Input: part model. Units: mm. Frame: model coordinates. A direction names the side the tool comes from. Round coordinates to 2 decimals unless told otherwise and drop trailing zeros. Loops run counter-clockwise (first coordinate to the right, second up) from the corner with the lowest first, then second, coordinate; pieces in that order, holes last. Notation, with made-up numbers: M 25.25,78 L 74.25,78 A15 cw 74.25,105 Z; hole C -22.75,17 d10. An arc over 180 degrees is marked long. Return JSON: item names as keys, results as strings. Group by question number.
1) Section C-C (x = 0). Output: boundary loops of the cut face in (y, z).
2) Mould query, pull axis Y, two halves, no side actions, for faces 1 (the face through (-13.851, 17.146, 8.479)), 2 (the face through (-24, 18, 9)), 3 (the face through (19.49, -11.72, 4.93)). Classes: +Y half, -Y half, draft (parallel to the pull), parting line (faces both ways), or undercut.
3) Material intervals for line 1 (Y direction, x = -7, z = 4.5); line 2 (X direction, y = 9, z = 9); line 3 (Y direction, x = -12, z = 3), sorted ascending. Write a range as from..to.
4) Contact query for flat-ended pins moving along their axis: P1, Ø3.5, axis at x = -12, y = 16, coming from the +Z side; P2, Ø1.5, axis at x = -1.5, z = 16.5, coming from the -Y side; P3, Ø12, axis at x = -12.5, z = 11.5, coming from the -Y side; P4, Ø1.5, axis at y = -10.5, z = 6, coming from the -X side. Output: stop coordinate, or through.
5) Section D-D (x = 7.5). Output: boundary loops of the cut face in (y, z).
6) Section A-A (y = 0). Output: boundary loops of the cut face in (x, z).
7) Access query for faces 4 (the face through (13.799, 10.824, 8.479)), 5 (the face through (-0.1, -7.8, 4.9)), 6 (the face through (0, -5, 4)), 7 (the face through (-19.72, -11.49, 4.93)), 8 (the face through (0, 25, 23)). Directions: +Z, -Z, +X, -X, +Y, -Y. A direction counts if a zero-diameter tool reaches every point of the face in a straight line with its end or side. Return the directions, or none.
8) Section B-B (z = 9). Count the separate pieces of the cut face and the enclosed holes in it, plus the area to 3 significant figures.
from build123d import *

# Parameters (mm, degrees)
PAD_DEPTH            = 24
POCKET_DEPTH         = 0.001
POCKET_DEPTH_BACK    = -32.001
SKETCH002_R          = 4.1
POCKET001_DEPTH      = 10.5
SKETCH003_R          = 2.25
HOLE_DEPTH           = 179.567934
POCKET002_DEPTH      = 172.567934
POCKET003_DEPTH      = 0.001
POCKET003_DEPTH_BACK = -32.001


with BuildPart() as part:
    # Sketch001 → Pad (new body, symmetric)
    with BuildSketch(Plane.YZ):
        Polygon((-16, 0), (-16, 10), (21, 10), (25, 14), (25, 32), (30, 32), (30, 0), align=None)
    extrude(amount=PAD_DEPTH, both=True)

    # Sketch → Pocket (cut, two sides)
    with BuildSketch(Plane.XY) as pocket_sk:
        with BuildLine():
            ThreePointArc((-15, 5), (-20, 0), (-15, -5))
            Line((-15, -5), (15, -5))
            ThreePointArc((15, -5), (20, 0), (15, 5))
            Line((15, 5), (-15, 5))
        make_face()
    extrude(amount=-POCKET_DEPTH, mode=Mode.SUBTRACT)
    extrude(pocket_sk.sketch, amount=-POCKET_DEPTH_BACK, mode=Mode.SUBTRACT)

    # Sketch002 → Pocket001 (cut, symmetric)
    with BuildSketch(Plane.XZ):
        with Locations((0, 9)):
            Circle(SKETCH002_R)
    extrude(amount=POCKET001_DEPTH, both=True, mode=Mode.SUBTRACT)

    # Sketch003 → Hole (cut, through all)
    with BuildSketch(Plane(origin=(12, 14, 0), x_dir=(1, 0, 0), z_dir=(0, 0, 1))):
        Circle(SKETCH003_R)
    hole = extrude(amount=HOLE_DEPTH, mode=Mode.SUBTRACT)

    # Sketch004 (on Sketch) → Pocket002 (cut, through all)
    with BuildSketch(Plane(origin=(12, 14, 7), x_dir=(1, 0, 0), z_dir=(0, 0, 1))):
        Polygon((0, 4.214657), (-3.65, 2.107328), (-3.65, -2.107328), (0, -4.214657), (3.65, -2.107328), (3.65, 2.107328), align=None)
    pocket002 = extrude(amount=POCKET002_DEPTH, mode=Mode.SUBTRACT)

    # Mirrored: Pocket002, Hole across YZ
    add(pocket002.mirror(Plane.YZ), mode=Mode.SUBTRACT)
    add(hole.mirror(Plane.YZ), mode=Mode.SUBTRACT)

    # Sketch005 → Pocket003 (cut, two sides)
    with BuildSketch(Plane.XY) as pocket003_sk:
        with BuildLine():
            ThreePointArc((-24, -1), (-19.606602, -11.606602), (-9, -16))
            Line((-9, -16), (9, -16))
            ThreePointArc((9, -16), (19.606602, -11.606602), (24, -1))
            Line((34, -1), (24, -1))
            Line((34, -1), (34, -69))
            Line((34, -69), (-34, -69))
            Line((-34, -69), (-34, -1))
            Line((-24, -1), (-34, -1))
        make_face()
    extrude(amount=-POCKET003_DEPTH, mode=Mode.SUBTRACT)
    extrude(pocket003_sk.sketch, amount=-POCKET003_DEPTH_BACK, mode=Mode.SUBTRACT)


solid = part.part
Returned:
{
 "1": {"outline": "M -16,0 L -5,0 L -5,4.9 L -10.5,4.9 L -10.5,10 L -16,10 Z; M 5,0 L 30,0 L 30,32 L 25,32 L 25,14 L 21,10 L 10.5,10 L 10.5,4.9 L 5,4.9 Z"},
 "2": {"face 1": "undercut", "face 2": "draft", "face 3": "-Y half"},
 "3": {"line 1": "y = -16..-5, 5..30", "line 2": "x = -24..-4.1, 4.1..24", "line 3": "y = -15.7..-5, 5..11.75, 16.25..30"},
 "4": {"P1": "stops at z = 7", "P2": "stops at y = 25", "P3": "stops at y = -16", "P4": "stops at x = -21.18"},
 "5": {"outline": "M -16,0 L -5,0 L -5,10 L -16,10 Z; M 5,0 L 30,0 L 30,32 L 25,32 L 25,14 L 21,10 L 5,10 Z"},
 "6": {"outline": "M -24,0 L -20,0 L -20,10 L -24,10 Z; M 20,0 L 24,0 L 24,10 L 20,10 Z"},
 "7": {"face 4": "+Z", "face 5": "none", "face 6": "+Z, -Z", "face 7": "+Z, -Z, -X, -Y", "face 8": "+Z, +X, -X, -Y"},
 "8": {"separate pieces": "1", "enclosed holes": "3", "area": "1,550 mm^2"}
}
